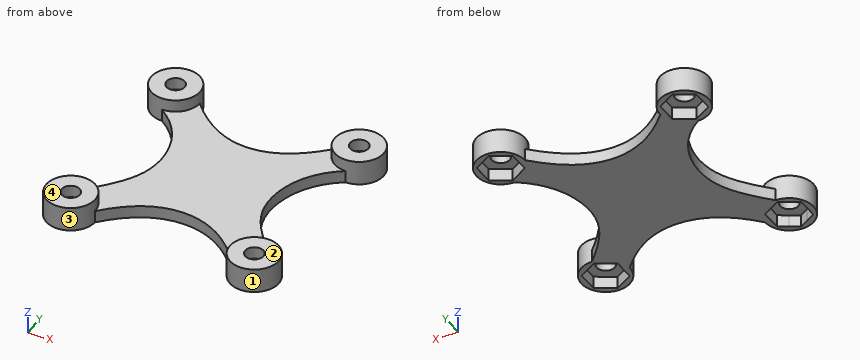
from build123d import *

# Parameters (mm, degrees)
F1_DEPTH = 2
F2_DEPTH = 4
F3_START = 2
F0_R     = 1.5
F3_DEPTH = 2


with BuildPart() as f1:
    # F0 (on Top) → F1 (new body)
    with BuildSketch(Plane.XY):
        with BuildLine():
            ThreePointArc((0, 4), (-2.8284271247, -2.8284271247), (4, 0))
            ThreePointArc((4, 0), (2.8284271247, 2.8284271247), (0, 4))
        make_face()
        Polygon((3, 1.7320508076), (3, 0), (3, -1.7320508076), (1.4999999564, -2.5980762365), (0, -3.4641016151), (-1.4999999973, -2.5980762129), (-3, -1.7320508076), (-3, 0), (-3, 1.7320508076), (-1.4999999564, 2.5980762365), (0, 3.4641016151), (1.4999999564, 2.5980762365), align=None, mode=Mode.SUBTRACT)
        with BuildLine():
            ThreePointArc((0, 4), (2.8284271247, 2.8284271247), (4, 0))
            add(Edge.make_bspline(
                [(4, 0), (7.75, 4.317717161), (15.25, 7.682282839), (22.75, 4.317717161), (26.5, 0)],
                knots=[0, 0, 0, 0, 0.5, 1, 1, 1, 1], degree=3))
            ThreePointArc((26.5, 0), (27.6715728753, 2.8284271247), (30.5, 4))
            add(Edge.make_bspline(
                [(30.5, 26.5), (25.9933560661, 23.4998809866), (22.921031967, 14.5143643781), (26.1645799999, 8.4713902573), (30.5, 4)],
                knots=[0, 0, 0, 0, 0.5, 1, 1, 1, 1], degree=3))
            ThreePointArc((30.5, 26.5), (27.6715728753, 27.6715728753), (26.5, 30.5))
            add(Edge.make_bspline(
                [(15.25, 24.5), (19, 24.5), (22.75, 26.3951093107), (26.5, 30.5)],
                knots=[0.5, 0.5, 0.5, 0.5, 1, 1, 1, 1], degree=3))
            add(Edge.make_bspline(
                [(4, 30.5), (7.75, 26.3951093107), (11.5, 24.5), (15.25, 24.5)],
                knots=[0, 0, 0, 0, 0.5, 0.5, 0.5, 0.5], degree=3))
            ThreePointArc((4, 30.5), (2.8284271247, 27.6715728753), (0, 26.5))
            add(Edge.make_bspline(
                [(0, 26.5), (4.5066439339, 23.4998809866), (7.578968033, 14.5143643781), (4.3354200001, 8.4713902573), (0, 4)],
                knots=[0, 0, 0, 0, 0.5, 1, 1, 1, 1], degree=3))
        make_face()
        with BuildLine():
            ThreePointArc((30.5, 4), (27.6715728753, 2.8284271247), (26.5, 0))
            ThreePointArc((26.5, 0), (30.5, -4), (34.5, 0))
            ThreePointArc((34.5, 0), (33.3284271247, 2.8284271247), (30.5, 4))
        make_face()
        Polygon((27.5, 1.7320508076), (30.5, 3.4641016151), (33.5, 1.7320508076), (33.5, -1.7320508076), (30.5, -3.4641016151), (27.5, -1.7320508076), align=None, mode=Mode.SUBTRACT)
        with BuildLine():
            ThreePointArc((4, 30.5), (-2.8284271247, 33.3284271247), (0, 26.5))
            ThreePointArc((0, 26.5), (2.8284271247, 27.6715728753), (4, 30.5))
        make_face()
        Polygon((-3, 32.2320508076), (0, 33.9641016151), (3, 32.2320508076), (3, 28.7679491924), (0, 27.0358983849), (-3, 28.7679491924), align=None, mode=Mode.SUBTRACT)
        with BuildLine():
            ThreePointArc((26.5, 30.5), (27.6715728753, 27.6715728753), (30.5, 26.5))
            ThreePointArc((30.5, 26.5), (33.3284271247, 27.6715728753), (34.5, 30.5))
            ThreePointArc((34.5, 30.5), (30.5, 34.5), (26.5, 30.5))
        make_face()
        Polygon((27.5, 32.2320508076), (30.5, 33.9641016151), (33.5, 32.2320508076), (33.5, 28.7679491924), (30.5, 27.0358983849), (27.5, 28.7679491924), align=None, mode=Mode.SUBTRACT)
    extrude(amount=F1_DEPTH)

    # F0 (on Top) → F2 (join)
    with BuildSketch(Plane.XY):
        with BuildLine():
            ThreePointArc((4, 30.5), (-2.8284271247, 33.3284271247), (0, 26.5))
            ThreePointArc((0, 26.5), (2.8284271247, 27.6715728753), (4, 30.5))
        make_face()
        Polygon((-3, 32.2320508076), (0, 33.9641016151), (3, 32.2320508076), (3, 28.7679491924), (0, 27.0358983849), (-3, 28.7679491924), align=None, mode=Mode.SUBTRACT)
        with BuildLine():
            ThreePointArc((26.5, 30.5), (27.6715728753, 27.6715728753), (30.5, 26.5))
            ThreePointArc((30.5, 26.5), (33.3284271247, 27.6715728753), (34.5, 30.5))
            ThreePointArc((34.5, 30.5), (30.5, 34.5), (26.5, 30.5))
        make_face()
        Polygon((27.5, 32.2320508076), (30.5, 33.9641016151), (33.5, 32.2320508076), (33.5, 28.7679491924), (30.5, 27.0358983849), (27.5, 28.7679491924), align=None, mode=Mode.SUBTRACT)
        with BuildLine():
            ThreePointArc((30.5, 4), (27.6715728753, 2.8284271247), (26.5, 0))
            ThreePointArc((26.5, 0), (30.5, -4), (34.5, 0))
            ThreePointArc((34.5, 0), (33.3284271247, 2.8284271247), (30.5, 4))
        make_face()
        Polygon((27.5, 1.7320508076), (30.5, 3.4641016151), (33.5, 1.7320508076), (33.5, -1.7320508076), (30.5, -3.4641016151), (27.5, -1.7320508076), align=None, mode=Mode.SUBTRACT)
        with BuildLine():
            ThreePointArc((0, 4), (-2.8284271247, -2.8284271247), (4, 0))
            ThreePointArc((4, 0), (2.8284271247, 2.8284271247), (0, 4))
        make_face()
        Polygon((3, 1.7320508076), (3, 0), (3, -1.7320508076), (1.4999999564, -2.5980762365), (0, -3.4641016151), (-1.4999999973, -2.5980762129), (-3, -1.7320508076), (-3, 0), (-3, 1.7320508076), (-1.4999999564, 2.5980762365), (0, 3.4641016151), (1.4999999564, 2.5980762365), align=None, mode=Mode.SUBTRACT)
    extrude(amount=F2_DEPTH)

    # F0 (on Top) → F3 (join)
    with BuildSketch(Plane.XY.offset(F3_START)):
        with BuildLine():
            ThreePointArc((1.4999999564, -2.5980762365), (2.5980761988, -1.5000000218), (3, 0))
            ThreePointArc((3, 0), (2.5980761988, 1.5000000218), (1.4999999564, 2.5980762365))
            ThreePointArc((1.4999999564, 2.5980762365), (0, 3), (-1.4999999564, 2.5980762365))
            ThreePointArc((-1.4999999564, 2.5980762365), (-2.5980761988, 1.5000000218), (-3, 0))
            ThreePointArc((-3, 0), (-2.5980762106, -1.5000000014), (-1.4999999973, -2.5980762129))
            ThreePointArc((-1.4999999973, -2.5980762129), (-2.36e-08, -3), (1.4999999564, -2.5980762365))
        make_face()
        Circle(F0_R, mode=Mode.SUBTRACT)
        with BuildLine():
            ThreePointArc((-3, 0), (-2.5980761988, 1.5000000218), (-1.4999999564, 2.5980762365))
            Line((-1.4999999564, 2.5980762365), (-3, 1.7320508076))
            Line((-3, 1.7320508076), (-3, 0))
        make_face()
        with BuildLine():
            ThreePointArc((1.4999999564, 2.5980762365), (2.5980761988, 1.5000000218), (3, 0))
            Line((3, 0), (3, 1.7320508076))
            Line((3, 1.7320508076), (1.4999999564, 2.5980762365))
        make_face()
        with BuildLine():
            Line((3, -1.7320508076), (3, 0))
            ThreePointArc((3, 0), (2.5980761988, -1.5000000218), (1.4999999564, -2.5980762365))
            Line((1.4999999564, -2.5980762365), (3, -1.7320508076))
        make_face()
        with BuildLine():
            Line((-3, -1.7320508076), (-1.4999999973, -2.5980762129))
            ThreePointArc((-1.4999999973, -2.5980762129), (-2.5980762106, -1.5000000014), (-3, 0))
            Line((-3, 0), (-3, -1.7320508076))
        make_face()
        with BuildLine():
            ThreePointArc((-1.4999999564, 2.5980762365), (0, 3), (1.4999999564, 2.5980762365))
            Line((1.4999999564, 2.5980762365), (0, 3.4641016151))
            Line((0, 3.4641016151), (-1.4999999564, 2.5980762365))
        make_face()
        with BuildLine():
            Line((0, -3.4641016151), (1.4999999564, -2.5980762365))
            ThreePointArc((1.4999999564, -2.5980762365), (-2.36e-08, -3), (-1.4999999973, -2.5980762129))
            Line((-1.4999999973, -2.5980762129), (0, -3.4641016151))
        make_face()
        Polygon((33.5, 1.7320508076), (30.5, 3.4641016151), (27.5, 1.7320508076), (27.5, -1.7320508076), (30.5, -3.4641016151), (33.5, -1.7320508076), align=None)
        with Locations((30.5, 0)):
            Circle(F0_R, mode=Mode.SUBTRACT)
        Polygon((33.5, 32.2320508076), (30.5, 33.9641016151), (27.5, 32.2320508076), (27.5, 28.7679491924), (30.5, 27.0358983849), (33.5, 28.7679491924), align=None)
        with Locations((30.5, 30.5)):
            Circle(F0_R, mode=Mode.SUBTRACT)
        Polygon((3, 32.2320508076), (0, 33.9641016151), (-3, 32.2320508076), (-3, 28.7679491924), (0, 27.0358983849), (3, 28.7679491924), align=None)
        with Locations((0, 30.5)):
            Circle(F0_R, mode=Mode.SUBTRACT)
    extrude(amount=F3_DEPTH)


solid = f1.part
Geometry check sheet. Reference: the model listing, model coordinates, mm. Face numbers are marked on the shaded views. A direction names the side the tool comes from. Coordinates: 2 decimals unless noted, no trailing zeros. Write each loop counter-clockwise with the first axis right and the second up, starting at its lowest first coordinate (ties: lowest second). Pieces come first, ordered by that corner, then holes. Notation, with made-up numbers: (48.25, 22) -> (52.25, 22) arc R27 ccw to (52.25, 38) -> close; hole circle Ø6 at (-40, 5). An arc over 180 degrees is marked (long way). One line per question, with ' | ' between items.
1. Set-up check for the marked faces 1 and 2: record each of +Z, -Z, +X, -X, +Y, -Y from which the full face is reachable in a straight line by a thin tool's end or side.
Answers:
face 1: +Z | face 2: +Z, +X, -X, +Y, -Y
2. Thickness scan on probe 1 along Y at (x, z) = (0, 3); probe 2 along X at (y, z) = (-2, 2.5); probe 3 along Y at (x, z) = (29, 0.6). Record the ranges inside material, lowest first. Write a range as from..to.
Answers:
probe 1: y = -4..-1.5, 1.5..4, 26.5..29, 32..34.5 | probe 2: x = -3.46..3.46, 27.04..33.96 | probe 3: y = -3.71..-2.6, 2.6..5.61, 25.36..27.9, 33.1..34.21
3. Cross-section at A-A on z = 3.1. Record the cut outline in (x, y), and give its area (3 significant figures).
Answers:
outline: circle Ø8 at (0, 0); circle Ø8 at (0, 30.5); circle Ø8 at (30.5, 0); circle Ø8 at (30.5, 30.5); hole circle Ø3 at (0, 0); hole circle Ø3 at (0, 30.5); hole circle Ø3 at (30.5, 0); hole circle Ø3 at (30.5, 30.5) | area: 173 mm²
4. Draft check along X on the marked faces 3 and 4. Enter one of: +X half, -X half, draft (parallel to the pull), parting line (faces both ways), or undercut.
Answers:
face 3: undercut | face 4: draft
5. Depth check by flat-ended pin: pin 1 Ø2.5 at (x, y) = (0, 30.5) entering from -Z; pin 2 Ø2 at (x, z) = (25, 2.5) entering from -Y (3 decimals); pin 3 Ø1 at (y, z) = (1, 0.5) entering from -X; pin 4 Ø2 at (x, z) = (11.5, 1.5) entering from -Y. Enter the tip coordinate at first touch or a pass-through.
Answers:
pin 1: passes through | pin 2: stops at y = 0.705 | pin 3: stops at x = -3.97 | pin 4: stops at y = 5.03
